Design review of the part built by this model. Coordinates are the model's own, in mm. Face numbers are marked on the shaded views. Give positions to 0.01 mm unless a question says otherwise; leave off trailing zeros. Order: outer loops, then holes, each group sorted by start corner. A loop starts at its lowest first (then second) coordinate and runs counter-clockwise, first axis right, second up. Notation, with made-up numbers: (7, -27) -> (46, -27) arc R24 cw to (46, 6) -> close; hole circle Ø10 at (-28, 13.25). An arc over 180 degrees is marked (long way). Use a Markdown table: item, result. Add a question column.
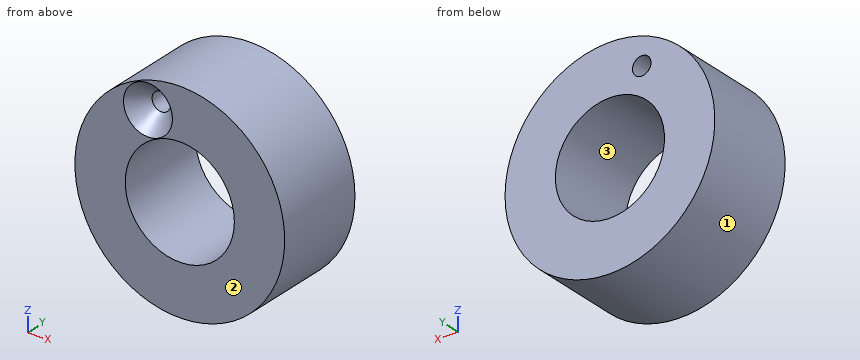
```python
from build123d import *

# Parameters (mm, degrees)
F0_R           = 28.9202335228
F1_DEPTH       = 25.4
F2_R           = 15.0449278179
F3_DEPTH       = 25.401
F5_D           = 5.1054
F5_CSINK_D     = 13.4874
F5_CSINK_ANGLE = 82


with BuildPart() as f1:
    # F0 (on Front) → F1 (new body)
    with BuildSketch(Plane.XZ):
        with Locations((24.1588130593, 38.0158424377)):
            Circle(F0_R)
    extrude(amount=F1_DEPTH)

    # F2 (on face) → F3 (cut, through all)
    with BuildSketch(Plane.XZ.offset(25.4)):
        with Locations((24.1588130593, 38.0158424377)):
            Circle(F2_R)
    extrude(amount=-F3_DEPTH, mode=Mode.SUBTRACT)

    # F5 (through all)
    with Locations(Plane.XZ.offset(25.4)):
        with Locations((15.3881106526, 58.0915510654)):
            CounterSinkHole(F5_D / 2, F5_CSINK_D / 2, counter_sink_angle=F5_CSINK_ANGLE)


solid = f1.part
```
1) Add section A-A (z = 24.5). Give the boundary of the cut face in (x, y).
2) For L1, parallel to Z at x = 24, y = -23; L2, parallel to Z at x = 20, y = -24; L3, parallel to X at y = -4, z = 57, list the stretches that pass through material, from the lowest coordinate up. Write a range as [from, to].
3) Add section B-B (x = 33.5). Give the boundary of the cut face in (y, z), then the cut area to 3 significant figures.
4) The part is to be moulded in two halves that separate along X. For the marked faces 1, 2 and 3, say which applies: +X half, -X half, draft (parallel to the pull), parting line (faces both ways), or undercut.
5) Add section C-C (y = -19.75). Give the boundary of the cut face in (x, z).
6) Insertion check: pin 1 (24 mm diameter, centred on x = 24.16, z = 38.02, fed in from +Y); pin 2 (5 mm diameter, centred on x = 47, y = -13.5, fed in from -Z); pin 3 (5 mm diameter, centred on x = 32.5, y = -15, fed in from +Z); pin 4 (3 mm diameter, centred on x = 43, y = -19.5, fed in from +Z). Each pin has a flat end and moves straight along its axis. Give the tip position at first contact, or say it passes through.
7) Add section D-D (x = 45). Give the boundary of the cut face in (y, z).
Worked answers:
| question | item | result |
|---|---|---|
| 1 | outline | (-1.41, -25.4) -> (17.55, -25.4) -> (17.55, 0) -> (-1.41, 0) -> close; (30.77, -25.4) -> (49.73, -25.4) -> (49.73, 0) -> (30.77, 0) -> close |
| 2 | L1 | [9.1, 22.97], [53.06, 66.94] |
| 2 | L2 | [9.4, 23.56], [52.47, 55.05], [61.14, 66.64] |
| 2 | L3 | [2.34, 13.08], [17.7, 45.98] |
| 3 | outline | (-25.4, 10.65) -> (0, 10.65) -> (0, 26.22) -> (-25.4, 26.22) -> close; (-25.4, 49.81) -> (0, 49.81) -> (0, 65.39) -> (-25.4, 65.39) -> close |
| 3 | area | 791 mm^2 |
| 4 | face 1 | parting line |
| 4 | face 2 | draft |
| 4 | face 3 | undercut |
| 5 | outline | circle Ø57.84 at (24.16, 38.02); hole circle Ø30.09 at (24.16, 38.02); hole circle Ø5.11 at (15.39, 58.09) |
| 6 | pin 1 | through |
| 6 | pin 2 | z = 17.46 |
| 6 | pin 3 | z = 66.34 |
| 6 | pin 4 | z = 61.16 |
| 7 | outline | (-25.4, 17.97) -> (0, 17.97) -> (0, 58.07) -> (-25.4, 58.07) -> close |
